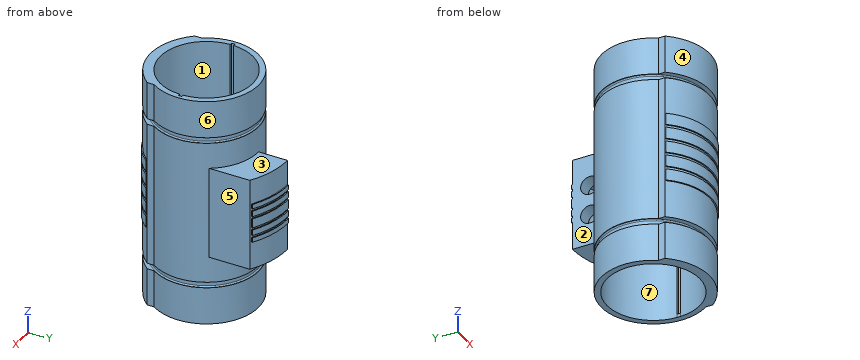
from build123d import *

# Parameters (mm, degrees)
ESBO_O1_R                     = 45
RESSALTO_EXTRUS_O1_DEPTH      = 200
ESBO_O2_R                     = 40
CORTE_EXTRUS_O2_DEPTH         = 200
RESSALTO_EXTRUS_O2_DEPTH      = 200
ESBO_O6_W                     = 10
ESBO_O6_H                     = 1
REVOLU_O1_ANGLE               = 50
REVOLU_O1_OTHER_WAY_ANGLE     = 50
RESSALTO_EXTRUS_O6_DEPTH      = 40
RESSALTO_EXTRUS_O6_DEPTH_BACK = 40
CORTE_EXTRUS_O3_DEPTH         = 12
CORTE_REVOLU_O5_ANGLE         = 180
ESBO_O20_W                    = 4
ESBO_O20_H                    = 1
ESBO_O20_W_2                  = 5
ESBO_O20_W_3                  = 8
REVOLU_O3_ANGLE               = 32
ESBO_O21_W                    = 2.028134895
ESBO_O21_H                    = 3
RESSALTO_EXTRUS_O8_DEPTH      = 3


with BuildPart() as part:
    # Esboço1 → Ressalto-extrusão1 (new body)
    with BuildSketch(Plane.XY):
        Circle(ESBO_O1_R)
    extrude(amount=RESSALTO_EXTRUS_O1_DEPTH)

    # Esboço2 → Corte-extrusão2 (cut)
    with BuildSketch(Plane.XY):
        Circle(ESBO_O2_R)
        Polygon((0, -1.5), (42, -1.5), (42, 1.5), (-42, 1.5), (-42, -1.5), align=None)
    extrude(amount=CORTE_EXTRUS_O2_DEPTH, mode=Mode.SUBTRACT)

    # Esboço4 → Ressalto-extrusão2 (add)
    with BuildSketch(Plane.XY):
        with BuildLine():
            Line((-37.5, -24.874685928), (-37.5, -30.757112998))
            ThreePointArc((-37.5, -30.757112998), (0, -48.5), (37.5, -30.757112998))
            Line((37.5, -30.757112998), (37.5, -24.874685928))
            ThreePointArc((37.5, -24.874685928), (36.193272903, -26.740362685), (34.793814433, -28.537527524))
            ThreePointArc((34.793814433, -28.537527524), (0, -45), (-34.793814433, -28.537527524))
            ThreePointArc((-34.793814433, -28.537527524), (-36.193272903, -26.740362685), (-37.5, -24.874685928))
        make_face()
    extrude(amount=RESSALTO_EXTRUS_O2_DEPTH)

    # Esboço6 → Revolução1 (revolve)
    with BuildSketch(Plane(origin=(0, 0, 0), x_dir=(0, 0, -1), z_dir=(1, 0, 0))):
        Polygon((-75, -48.5), (-80, -48.5), (-80, -49.5), (-70, -49.5), (-70, -48.5), align=None)
        Polygon((-105, -49.5), (-105, -48.5), (-100, -48.5), (-95, -48.5), (-95, -49.5), align=None)
        with Locations((-125, -49)):
            Rectangle(ESBO_O6_W, ESBO_O6_H)
        Polygon((-92.5, -49.5), (-82.5, -49.5), (-82.5, -48.5), (-87.5, -48.5), (-92.5, -48.5), align=None)
        with Locations((-112.5, -49)):
            Rectangle(ESBO_O6_W, ESBO_O6_H)
    revolve(axis=Axis((0, 0, 0), (0, 0, 1)), revolution_arc=REVOLU_O1_ANGLE)

    # Esboço6 → Revolução1 other way (revolve)
    with BuildSketch(Plane(origin=(0, 0, 0), x_dir=(0, 0, -1), z_dir=(1, 0, 0))):
        Polygon((-75, -48.5), (-80, -48.5), (-80, -49.5), (-70, -49.5), (-70, -48.5), align=None)
        Polygon((-105, -49.5), (-105, -48.5), (-100, -48.5), (-95, -48.5), (-95, -49.5), align=None)
        with Locations((-125, -49)):
            Rectangle(ESBO_O6_W, ESBO_O6_H)
        Polygon((-92.5, -49.5), (-82.5, -49.5), (-82.5, -48.5), (-87.5, -48.5), (-92.5, -48.5), align=None)
        with Locations((-112.5, -49)):
            Rectangle(ESBO_O6_W, ESBO_O6_H)
    revolve(axis=Axis((0, 0, 0), (0, 0, -1)), revolution_arc=REVOLU_O1_OTHER_WAY_ANGLE)

    # Esboço7 → Corte-Revolução3 (revolve, cut)
    with BuildSketch(Plane(origin=(0, 0, 0), x_dir=(0, 0, -1), z_dir=(1, 0, 0)), mode=Mode.PRIVATE) as corte_revolu_o3_sk:
        with BuildLine():
            Line((-165, -48.5), (-162.5, -48.5))
            Line((-162.5, -48.5), (-162.5, -47.198708602))
            Line((-162.5, -47.198708602), (-162.5, -44.5))
            ThreePointArc((-162.5, -44.5), (-162.792893219, -43.792893219), (-163.5, -43.5))
            Line((-163.5, -43.5), (-166.5, -43.5))
            ThreePointArc((-166.5, -43.5), (-167.207106781, -43.792893219), (-167.5, -44.5))
            Line((-167.5, -44.5), (-167.5, -48.5))
            Line((-167.5, -48.5), (-165, -48.5))
        make_face()
        with BuildLine():
            Line((-37.5, -48.5), (-37.5, -44.5))
            ThreePointArc((-37.5, -44.5), (-37.207106781, -43.792893219), (-36.5, -43.5))
            Line((-36.5, -43.5), (-33.5, -43.5))
            ThreePointArc((-33.5, -43.5), (-32.792893219, -43.792893219), (-32.5, -44.5))
            Line((-32.5, -44.5), (-32.5, -47.198708602))
            Line((-32.5, -47.198708602), (-32.5, -48.5))
            Line((-32.5, -48.5), (-37.5, -48.5))
        make_face()
    revolve(corte_revolu_o3_sk.sketch.rotate(Axis((0, 0, 0), (0, 0, 1)), 270), axis=Axis((0, 0, 0), (0, 0, 1)), mode=Mode.SUBTRACT)

    # Esboço17 → Ressalto-extrusão6 (add, two sides: drawn at the far end of the back side and taken through both)
    with BuildSketch(Plane(origin=(0, 0, 100), x_dir=(-1, 0, 0), z_dir=(0, 0, -1)).offset(-RESSALTO_EXTRUS_O6_DEPTH_BACK)):
        with BuildLine():
            Line((0, 45), (0, 70))
            ThreePointArc((0, 70), (-20.056825735, 67.065070949), (-38.431784027, 58.506392612))
            Line((-38.431784027, 58.506392612), (-38.431784027, 23.409356601))
            ThreePointArc((-38.431784027, 23.409356601), (-22.040632397, 39.23277359), (0, 45))
        make_face()
    extrude(amount=RESSALTO_EXTRUS_O6_DEPTH + RESSALTO_EXTRUS_O6_DEPTH_BACK)

    # Esboço18 → Corte-extrusão3 (cut)
    with BuildSketch(Plane(origin=(0, 0, 0), x_dir=(0, 0, -1), z_dir=(1, 0, 0))):
        with BuildLine():
            ThreePointArc((-95, 55), (-87, 47), (-79, 55))
            Line((-79, 55), (-95, 55))
        make_face()
        with BuildLine():
            Line((-95, 55), (-79, 55))
            ThreePointArc((-79, 55), (-87, 63), (-95, 55))
        make_face()
        with BuildLine():
            ThreePointArc((-121, 55), (-113, 47), (-105, 55))
            Line((-105, 55), (-121, 55))
        make_face()
        with BuildLine():
            Line((-121, 55), (-105, 55))
            ThreePointArc((-105, 55), (-113, 63), (-121, 55))
        make_face()
    extrude(amount=CORTE_EXTRUS_O3_DEPTH, mode=Mode.SUBTRACT)

    # Esboço19 → Corte-Revolução5 (revolve, cut)
    with BuildSketch(Plane.ZY.offset(-12)):
        Polygon((100, 45), (77.5, 45), (77.5, 65), (122.5, 65), (122.5, 45), align=None)
    revolve(axis=Axis((12, 45, 100), (0, 0, -1)), revolution_arc=CORTE_REVOLU_O5_ANGLE, mode=Mode.SUBTRACT)

    # Esboço20 → Revolução3 (revolve)
    with BuildSketch(Plane(origin=(0, 0, 0), x_dir=(0, 0, -1), z_dir=(1, 0, 0))):
        with Locations((-86.242439745, 70.5)):
            Rectangle(ESBO_O20_W, ESBO_O20_H)
        with Locations((-92.742439745, 70.5)):
            Rectangle(ESBO_O20_W_2, ESBO_O20_H)
        with Locations((-101.242439745, 70.5)):
            Rectangle(ESBO_O20_W_3, ESBO_O20_H)
        with Locations((-109.742439745, 70.5)):
            Rectangle(ESBO_O20_W_2, ESBO_O20_H)
        with Locations((-116.242439745, 70.5)):
            Rectangle(ESBO_O20_W, ESBO_O20_H)
    revolve(axis=Axis((0, 0, 0), (0, 0, -1)), revolution_arc=REVOLU_O3_ANGLE)

    # Esboço21 → Ressalto-extrusão8 (add)
    with BuildSketch(Plane.XY):
        with Locations((40.985932553, 0)):
            Rectangle(ESBO_O21_W, ESBO_O21_H)
        with Locations((-40.985932553, 0)):
            Rectangle(ESBO_O21_W, ESBO_O21_H)
    extrude(amount=RESSALTO_EXTRUS_O8_DEPTH)


solid = part.part
Here's how the part is built. I have some questions about the finished solid (model axes, mm). Face numbers are marked on the shaded views. A direction names the side the tool comes from. Give positions to 0.01 mm unless a question says otherwise; leave off trailing zeros. Loops run counter-clockwise (first coordinate to the right, second up) from the corner with the lowest first, then second, coordinate; pieces in that order, holes last. Notation, with made-up numbers: (3.5, -13) -> (48.5, -13) arc R27 ccw to (48.5, 8) -> close; hole circle Ø11 at (-13.75, -39.75). An arc over 180 degrees is marked (long way). Answer as a JSON object with one key per item and string values. Group by question number.
Item 1: On a 3-axis mill with a long thin cutter (end or side, diameter ignored), from which of +Z, -Z, +X, -X, +Y, -Y can I reach the whole of each face in a straight line? I mean the marked faces 1, 2, 3 and 4. Say none if no direction works.
Item 2: Imagine slicing it at A-A on z = 158.5. Write out the boundary of the cut face in (x, y).
Item 3: Will these pins go through, and if not, where does the flat tip stop? pin 1 (1 mm diameter, centred on y = -15.5, z = 175.5, fed in from +X); pin 2 (3 mm diameter, centred on y = -29, z = 177.5, fed in from +X); pin 3 (13.5 mm diameter, centred on y = 46.5, z = 106.5, fed in from +X); pin 4 (6 mm diameter, centred on x = 33, y = -17, fed in from +Z).
Item 4: Thinking about a two-plate mould opening in X: for the marked faces 5, 6 and 7, which applies, pulls with the +X half, pulls with the -X half, needs draft (parallel to the pull), parting line crosses it, or undercut?
Item 5: I need wall thicknesses on L1, parallel to Z at x = 31, y = 47; L2, parallel to Y at x = 7, z = 113; L3, parallel to Y at x = 5, z = 113. Which ranges of each line are inside material? Lowest first, please.
Item 6: Imagine slicing it at B-B on z = 137. Write out the boundary of the cut face in (x, y), then the cut area to 3 significant figures.
Answer list:
{
 "1": {"face 1": "+Z, -Z", "face 2": "+Z, -Z, -X, +Y", "face 3": "+Z, +X, +Y", "face 4": "+Z, -Y"},
 "2": {"outline": "(-37.5, -30.76) arc R48.5 ccw to (37.5, -30.76) -> (37.5, -24.87) arc R45 ccw (long way) to (-37.5, -24.87) -> close; hole (-42, -1.5) -> (-39.97, -1.5) arc R40 ccw to (39.97, -1.5) -> (42, -1.5) -> (42, 1.5) -> (39.97, 1.5) arc R40 ccw to (-39.97, 1.5) -> (-42, 1.5) -> close"},
 "3": {"pin 1": "stops at x = 42.43", "pin 2": "stops at x = 37.5", "pin 3": "stops at x = 38.43", "pin 4": "stops at z = 200"},
 "4": {"face 5": "pulls with the +X half", "face 6": "parting line crosses it", "face 7": "undercut"},
 "5": {"L1": "z = 60 to 77.5, 122.5 to 140", "L2": "y = -49 to -39.38, 39.38 to 47, 63 to 69.65", "L3": "y = -49.25 to -39.69, 39.69 to 47, 63 to 69.82"},
 "6": {"outline": "(-37.5, -30.76) arc R48.5 ccw to (37.5, -30.76) -> (37.5, -24.87) arc R45 ccw to (38.43, 23.41) -> (38.43, 58.51) arc R70 ccw to (0, 70) -> (0, 45) arc R45 ccw to (-37.5, -24.87) -> close; hole (-42, -1.5) -> (-39.97, -1.5) arc R40 ccw to (39.97, -1.5) -> (42, -1.5) -> (42, 1.5) -> (39.97, 1.5) arc R40 ccw to (-39.97, 1.5) -> (-42, 1.5) -> close", "area": "2,690 mm2"}
}
